from build123d import *

# Parameters (mm, degrees)
F0_W     = 100
F0_H     = 60
F1_DEPTH = 60
F2_W     = 40
F2_H     = 20
F3_DEPTH = 60.001
F4_W     = 20
F4_H     = 20
F5_DEPTH = 100.001
F6_W     = 60
F6_H     = 20
F7_DEPTH = 60.001
F8_W     = 20
F8_H     = 20
F9_DEPTH = 100.001


with BuildPart() as f1:
    # F0 (on Top) → F1 (new body)
    with BuildSketch(Plane.XY):
        with Locations((50, -30)):
            Rectangle(F0_W, F0_H)
    extrude(amount=F1_DEPTH)

    # F2 (on face) → F3 (cut, through all)
    with BuildSketch(Plane(origin=(0, 0, 0), x_dir=(1, 0, 0), z_dir=(0, 0, -1))):
        with Locations((80, 50)):
            Rectangle(F2_W, F2_H)
    extrude(amount=-F3_DEPTH, mode=Mode.SUBTRACT)

    # F4 (on face) → F5 (cut, through all)
    with BuildSketch(Plane.YZ.offset(100)):
        with Locations((-10, 30)):
            Rectangle(F4_W, F4_H)
    extrude(amount=-F5_DEPTH, mode=Mode.SUBTRACT)

    # F6 (on face) → F7 (cut, through all)
    with BuildSketch(Plane.XY.offset(60)):
        with Locations((30, -10)):
            Rectangle(F6_W, F6_H)
    extrude(amount=-F7_DEPTH, mode=Mode.SUBTRACT)

    # F8 (on face) → F9 (cut, through all)
    with BuildSketch(Plane(origin=(0, 0, 0), x_dir=(0, -1, 0), z_dir=(-1, 0, 0))):
        with Locations((50, 30)):
            Rectangle(F8_W, F8_H)
    extrude(amount=-F9_DEPTH, mode=Mode.SUBTRACT)


solid = f1.part
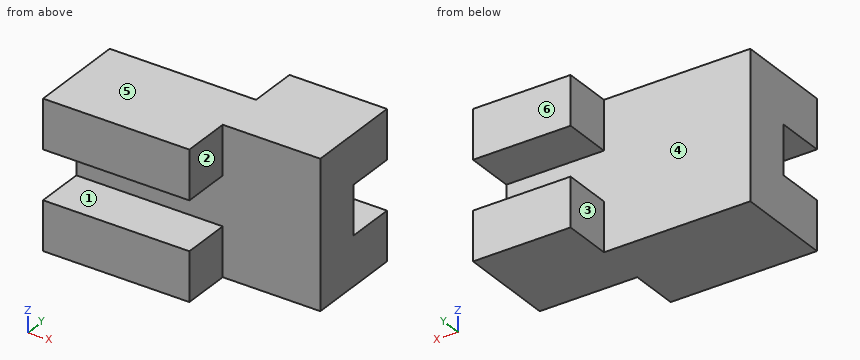
Design review of the part built by this model. Coordinates are the model's own, in mm. Face numbers are marked on the shaded views. A direction names the side the tool comes from. Coordinates: 2 decimals unless noted, no trailing zeros. Order: outer loops, then holes, each group sorted by start corner. A loop starts at its lowest first (then second) coordinate and runs counter-clockwise, first axis right, second up. Notation, with made-up numbers: (-17.5, 61) -> (20.5, 61) arc R7 ccw to (20.5, 71) -> close; hole circle Ø10 at (12.5, -39.75). An arc over 180 degrees is marked (long way). Use one line per item in the form item = value. Start each with the question number.
(1) Add section D-D on y = -12. State the section outline as (x, z) points, plus the area to 3 significant figures.
(2) The part is to be moulded in two halves that separate along Z. For the marked faces 4, 5 and 6, say which applies: +Z half, -Z half, draft (parallel to the pull), parting line (faces both ways), or undercut.
(3) Insertion check: pin 1 (10 mm diameter, centred on y = -7, z = 46, fed in from -X); pin 2 (16 mm diameter, centred on y = -54, z = 14.5, fed in from +X). Each pin has a flat end and moves straight along its axis. Give the tip position at first contact, or say it passes through.
(4) For the marked faces 1, 2 and 3, list the 3-axis set-ups (+Z, -Z, +X, -X, +Y, -Y) from which the entire face can be reached by the end or side of a thin tool; tool diameter is ignored.
(5) Add section A-A on y = -49.5. State the section outline as (x, z) points.
(6) Add section C-C on z = 47. State the section outline as (x, y) points.
(7) Add section B-B on x = 9. State the section outline as (y, z) points, plus the area to 3 significant figures.
(8) For probe 1 along Z at (x, y) = (69, -18); probe 2 along X at (y, z) = (-47, 9.5); probe 3 along Y at (x, z) = (94, 56.5), list the stretches that pass through material, from the lowest coordinate up.
Answer block:
q1.outline = (60, 0) -> (100, 0) -> (100, 20) -> (60, 20) -> close; (60, 40) -> (100, 40) -> (100, 60) -> (60, 60) -> close
q1.area = 1,600 mm²
q2.face_4 = undercut
q2.face_5 = +Z half
q2.face_6 = draft
q3.pin_1 = 60
q3.pin_2 = 60
q4.face_1 = +X, -X, -Y
q4.face_2 = +Z, -Z, +X, -Y
q4.face_3 = +Z, -Z, -X, +Y
q5.outline = (0, 0) -> (60, 0) -> (60, 20) -> (0, 20) -> close; (0, 40) -> (60, 40) -> (60, 60) -> (0, 60) -> close
q6.outline = (0, -60) -> (60, -60) -> (60, -40) -> (100, -40) -> (100, 0) -> (60, 0) -> (60, -20) -> (0, -20) -> close
q7.outline = (-60, 0) -> (-20, 0) -> (-20, 60) -> (-60, 60) -> (-60, 40) -> (-40, 40) -> (-40, 20) -> (-60, 20) -> close
q7.area = 2,000 mm²
q8.probe_1 = 0 to 20, 40 to 60
q8.probe_2 = 0 to 60
q8.probe_3 = -40 to 0
